from build123d import *

# Parameters (mm, degrees)
F0_W     = 50
F0_H     = 8
F1_DEPTH = 2


with BuildPart() as f1:
    # F0 (on Front) → F1 (new body, symmetric)
    with BuildSketch(Plane.XZ):
        Polygon((31.9974, -5.5436906666), (31.9974, 8.5436906666), (-31.9974, 8.5436906666), (-31.9974, -8.5436906666), (-25.9974, -8.5436906666), (-25.9974, -5.5436906666), align=None)
        with Locations((-0.9974, 1.4563093334)):
            Rectangle(F0_W, F0_H, mode=Mode.SUBTRACT)
    extrude(amount=F1_DEPTH, both=True)


solid = f1.part
Read the model definition and answer for the solid it produces. Units are mm, in the model's axes. A direction names the side the tool comes from. Coordinates: 2 decimals unless noted, no trailing zeros. Loops run counter-clockwise (first coordinate to the right, second up) from the corner with the lowest first, then second, coordinate; pieces in that order, holes last.
Q1. The part is cut by section B-B on z = -1.25. Write down the section's boundary in (x, y), and give its area (3 significant figures).
Q2. The mould has two halves that part along Z. Classify faces 1 (the face through (-29, 0, -8.544)), 2 (the face through (-31.997, 0, 0)), 3 (the face through (24.003, 0, 1)): +Z half, -Z half, draft (parallel to the pull), parting line (faces both ways), or undercut.
Q3. The part is cut by section C-C on y = -1.45. Write down the section's boundary in (x, z).
Q4. Which of the six approach directions +Z, -Z, +X, -X, +Y, -Y give full straight-line access (tool end or side, diameter ignored) to faces 4 (the face through (-1, 0, -2.544)), 5 (the face through (0, 0, 8.544)), 6 (the face through (3, 0, -5.544))?
Q5. This flat-tipped pin is pushed along its axis until it touches: pin 1 Ø1.2 at (x, y) = (0.5, 1) entering from -Z. Where does it stop, or does it pass through?
Q6. The part is cut by section A-A on x = -14. Write down the section's boundary in (y, z).
Q7. Consider probe 1 along Z at (x, y) = (-19, -1.3); probe 2 along X at (y, z) = (1.35, -2); probe 3 along X at (y, z) = (0.35, -6.75). Determine where each line is inside the solid, lowest interval first.
Results below:
1. outline: (-32, -2) - (-26, -2) - (-26, 2) - (-32, 2) - close; (24, -2) - (32, -2) - (32, 2) - (24, 2) - close
1. area: 56.0 mm2
2. face 1: -Z half
2. face 2: draft
2. face 3: undercut
3. outline: (-32, -8.54) - (-26, -8.54) - (-26, -5.54) - (32, -5.54) - (32, 8.54) - (-32, 8.54) - close; hole (-26, -2.54) - (24, -2.54) - (24, 5.46) - (-26, 5.46) - close
4. face 4: +Y, -Y
4. face 5: +Z, +X, -X, +Y, -Y
4. face 6: -Z, +X, +Y, -Y
5. pin 1: stops at z = -5.54
6. outline: (-2, -5.54) - (2, -5.54) - (2, -2.54) - (-2, -2.54) - close; (-2, 5.46) - (2, 5.46) - (2, 8.54) - (-2, 8.54) - close
7. probe 1: z = -5.54 to -2.54, 5.46 to 8.54
7. probe 2: x = -32 to -26, 24 to 32
7. probe 3: x = -32 to -26
